from build123d import *

# Parameters (mm, degrees)
F0_R     = 14.1859
F1_DEPTH = 14.4018
F2_SIZE  = 4.445
F3_R     = 1.5875


# Not quite as in the source:
# - a feature names something its author has since deleted; it is built from what else it names


with BuildPart() as f1:
    # F0 (on Top) → F1 (new body)
    with BuildSketch(Plane.XY):
        Circle(F0_R)
        Polygon((-7.366, 0), (-3.683, 6.3791431243), (3.683, 6.3791431243), (7.366, 0), (3.683, -6.3791431243), (-3.683, -6.3791431243), align=None, mode=Mode.SUBTRACT)
    extrude(amount=F1_DEPTH)

    # F2
    f2_edges = [f1.edges().sort_by_distance(p)[0] for p in [
        (-14.1859, 0, 14.4018),
    ]]
    chamfer(f2_edges, length=F2_SIZE)

    # F3
    f3_edges = [f1.edges().sort_by_distance(p)[0] for p in [
        (-9.7409, 0, 14.4018),
        (-14.1859, 0, 9.9568),
    ]]
    fillet(f3_edges, radius=F3_R)


solid = f1.part
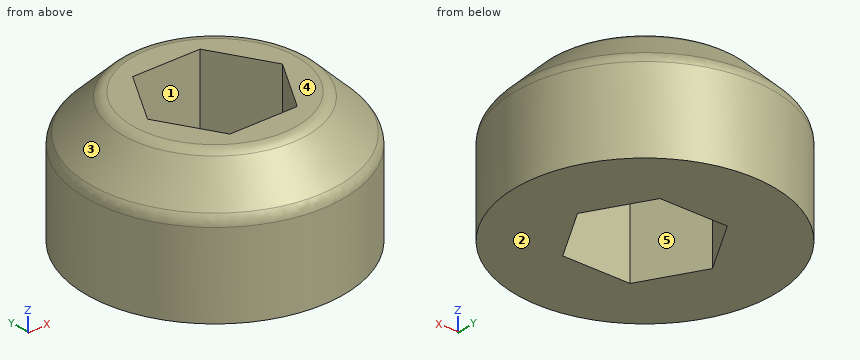
Check sheet for the modelled part. Datum: model origin and axes. Units: mm. Face numbers are marked on the shaded views. A direction names the side the tool comes from. Round coordinates to 2 decimals unless told otherwise and drop trailing zeros. Order: outer loops, then holes, each group sorted by start corner. A loop starts at its lowest first (then second) coordinate and runs counter-clockwise, first axis right, second up.
(1) Draft check along Y on the marked faces 3, 4 and 5. Enter one of: pulls with the +Y half, pulls with the -Y half, needs draft (parallel to the pull), parting line crosses it, or undercut.
(2) Cross-section at B-B, the plane z = 13.25. Enter the section's corners in (x, y), and give its area (3 significant figures).
(3) Go/stop test with flat-tipped pins: P1, Ø1, axis at x = 10.5, z = 7, coming from the +Y side; P2, Ø2, axis at y = -1.5, z = 4.5, coming from the +X side; P3, Ø1, axis at x = -9.5, y = -4.5, coming from the +Z side. Record where each tip stops, or that it passes through.
(4) Cross-section at A-A, the plane z = 5. Enter the section's corners in (x, y), and give its area (3 significant figures).
(5) Scan lines: probe 1 along X at (y, z) = (5.75, 6.75); probe 2 along Y at (x, z) = (4.75, 1); probe 3 along X at (y, z) = (-0.75, 7.5). Record each from-to range of solid material in increasing order.
(6) Access from +Z, -Z, +X, -X, +Y, -Y to the whole of each face (thin tool, end or side, straight path). Record for the marked faces 1 and 2.
Check sheet entries:
1. face 3: parting line crosses it
1. face 4: needs draft
1. face 5: undercut
2. outline: circle Ø21.79 at (0, 0); hole (-7.37, 0) - (-3.68, -6.38) - (3.68, -6.38) - (7.37, 0) - (3.68, 6.38) - (-3.68, 6.38) - close
2. area: 232 mm2
3. P1: stops at y = 10.06
3. P2: stops at x = 14.18
3. P3: stops at z = 14.1
4. outline: circle Ø28.37 at (0, 0); hole (-7.37, 0) - (-3.68, -6.38) - (3.68, -6.38) - (7.37, 0) - (3.68, 6.38) - (-3.68, 6.38) - close
4. area: 491 mm2
5. probe 1: x = -12.97 to -4.05, 4.05 to 12.97
5. probe 2: y = -13.37 to -4.53, 4.53 to 13.37
5. probe 3: x = -14.17 to -6.93, 6.93 to 14.17
6. face 1: +Z, -Z
6. face 2: -Z, +X, -X, +Y, -Y
